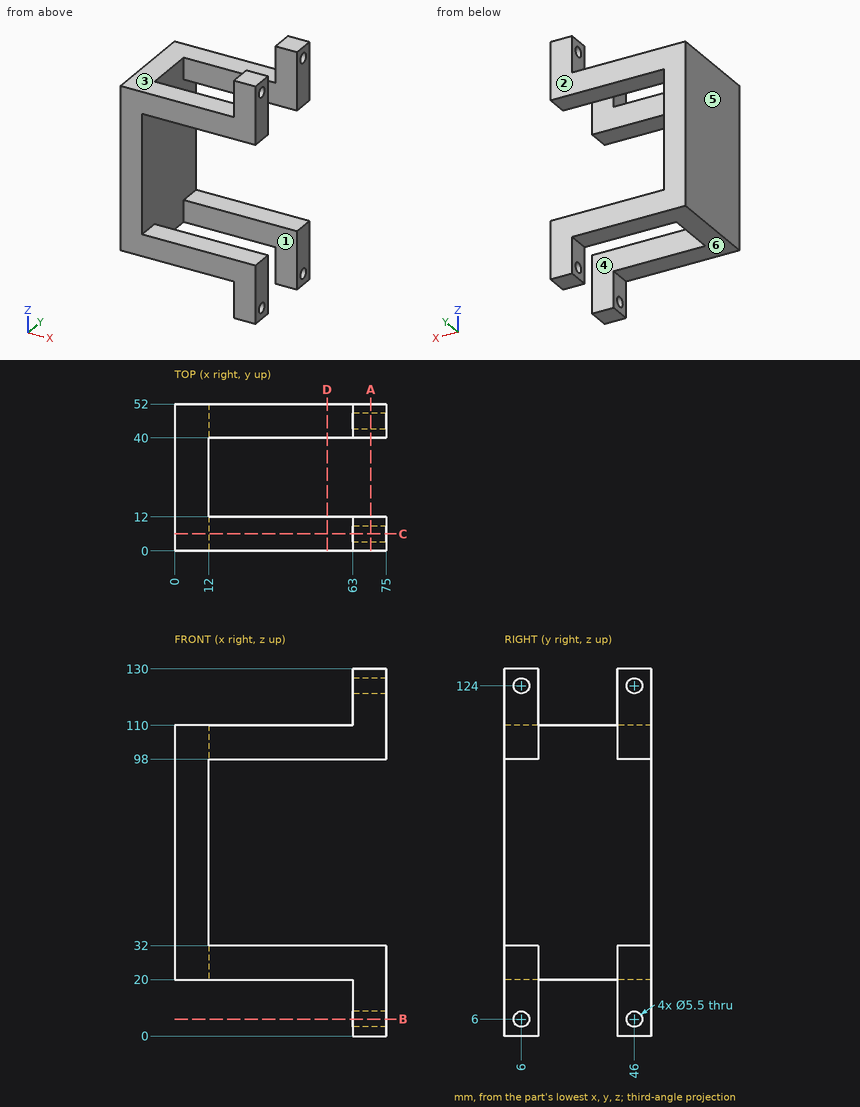
Could you check a few things on this drawing? It's one solid part, dimensions in mm from its lowest x, y, z. A direction names the side the tool comes from. Give positions to 0.01 mm unless a question says otherwise; leave off trailing zeros. Write each loop counter-clockwise with the first axis right and the second up, starting at its lowest first coordinate (ties: lowest second). Pieces come first, ordered by that corner, then holes. Notation, with made-up numbers: (77, 82.5) -> (115, 82.5) arc R27 ccw to (115, 109.5) -> close; hole circle Ø11 at (65, 27.5). An arc over 180 degrees is marked (long way). Write item = value, one per line.
(1) Suppose I cut it at C-C on y = 6. Write out the boundary of the cut face in (x, z), then the cut area to 3 significant figures.
Worked out:
outline = (0, 20) -> (63, 20) -> (63, 8.75) -> (75, 8.75) -> (75, 32) -> (12, 32) -> (12, 98) -> (75, 98) -> (75, 121.25) -> (63, 121.25) -> (63, 110) -> (0, 110) -> close; (63, 0) -> (75, 0) -> (75, 3.25) -> (63, 3.25) -> close; (63, 126.75) -> (75, 126.75) -> (75, 130) -> (63, 130) -> close
area = 2,940 mm^2
(2) Suppose I cut it at A-A on x = 69.5. Write out the boundary of the cut face in (y, z).
Worked out:
outline = (0, 0) -> (12, 0) -> (12, 32) -> (0, 32) -> close; (0, 98) -> (12, 98) -> (12, 130) -> (0, 130) -> close; (40, 0) -> (52, 0) -> (52, 32) -> (40, 32) -> close; (40, 98) -> (52, 98) -> (52, 130) -> (40, 130) -> close; hole circle Ø5.5 at (6, 6); hole circle Ø5.5 at (6, 124); hole circle Ø5.5 at (46, 6); hole circle Ø5.5 at (46, 124)
(3) I need wall thicknesses on probe 1 along Z at (x, y) = (67.75, 6); probe 2 along Z at (x, y) = (33.5, 5.5); probe 3 along Y at (x, z) = (29, 105). Which ranges of each line are inside material? Lowest first, please. Write a range as from..to.
Worked out:
probe_1 = 0..3.25, 8.75..32, 98..121.25, 126.75..130
probe_2 = 20..32, 98..110
probe_3 = 0..12, 40..52
(4) For the marked faces 4, 5 and 6, which set-ups out of +Z, -Z, +X, -X, +Y, -Y let a thin tool reach every point of the face, with its end or its side?
Worked out:
face_4 = +Z, -Z, +X
face_5 = +Z, -Z, -X, +Y, -Y
face_6 = -Z, -X, +Y, -Y
(5) Suppose I cut it at D-D on x = 54. Write out the boundary of the cut face in (y, z), then the cut area to 3 significant figures.
Worked out:
outline = (0, 20) -> (12, 20) -> (12, 32) -> (0, 32) -> close; (0, 98) -> (12, 98) -> (12, 110) -> (0, 110) -> close; (40, 20) -> (52, 20) -> (52, 32) -> (40, 32) -> close; (40, 98) -> (52, 98) -> (52, 110) -> (40, 110) -> close
area = 576 mm^2
(6) I'm going to push flat-ended pins straight in: P1, Ø3, axis at y = 21.5, z = 73.5, coming from the +X side; P2, Ø9.5, axis at y = 44, z = 119, coming from the -X side; P3, Ø9.5, axis at x = 43.5, y = 7, coming from the +Z side. Where does each tip first touch, or does it pass through?
Worked out:
P1 = 12
P2 = 63
P3 = 110
(7) Thinking about a two-plate mould opening in Y: for the marked faces 1, 2 and 3, which applies, released by +Y, released by -Y, zero draft, split by the parting line, or undercut?
Worked out:
face_1 = undercut
face_2 = released by +Y
face_3 = zero draft
(8) Suppose I cut it at B-B on z = 6. Write out the boundary of the cut face in (x, y).
Worked out:
outline = (63, 0) -> (75, 0) -> (75, 3.25) -> (63, 3.25) -> close; (63, 8.75) -> (75, 8.75) -> (75, 12) -> (63, 12) -> close; (63, 40) -> (75, 40) -> (75, 43.25) -> (63, 43.25) -> close; (63, 48.75) -> (75, 48.75) -> (75, 52) -> (63, 52) -> close
